Could you check a few things on this model? Use its own coordinates, in mm. Face numbers are marked on the shaded views. A direction names the side the tool comes from. Give positions to 0.01 mm unless a question says otherwise; leave off trailing zeros. Write each loop counter-clockwise with the first axis right and the second up, starting at its lowest first coordinate (ties: lowest second). Pieces come first, ordered by that corner, then holes. Notation, with made-up numbers: (47.5, 45) - (104.5, 45) arc R17 ccw to (104.5, 64) - close; hole circle Ø10 at (-14, -5.5). An arc over 180 degrees is marked (long way). Answer as CSV lines item,"result". Start each with the question number.
Q1. Imagine slicing it at A-A on z = 1.75. List the corners of the cut face in (x, y) for me, and give its area (3 significant figures).
Q2. Will these pins go through, and if not, where does the flat tip stop? pin 1 Ø1.5 at (x, z) = (52, 7.5) entering from -Y; pin 2 Ø3.5 at (y, z) = (6, 6) entering from -X; pin 3 Ø5 at (x, y) = (11.5, 38) entering from +Z.
Q3. Imagine slicing it at B-B on x = 33.5. List the corners of the cut face in (y, z) for me.
Q4. Imagine slicing it at C-C on y = 47.5. List the corners of the cut face in (x, z) for me, and give its area (3 significant figures).
Q5. Imagine slicing it at D-D on z = 8. List the corners of the cut face in (x, y) for me, and give its area (3 significant figures).
Q6. If I drill on line 1 along Y through (x, z) = (54.75, 6); line 2 along Z through (x, y) = (45.5, 21); line 3 along X through (y, z) = (11.5, 7), over which ranges is the centre line in solid material (lowest first)?
Q7. On a 3-axis mill with a long thin cutter (end or side, diameter ignored), from which of +Z, -Z, +X, -X, +Y, -Y can I reach the whole of each face in a straight line? I mean the marked faces 1 and 2. Say none if no direction works.
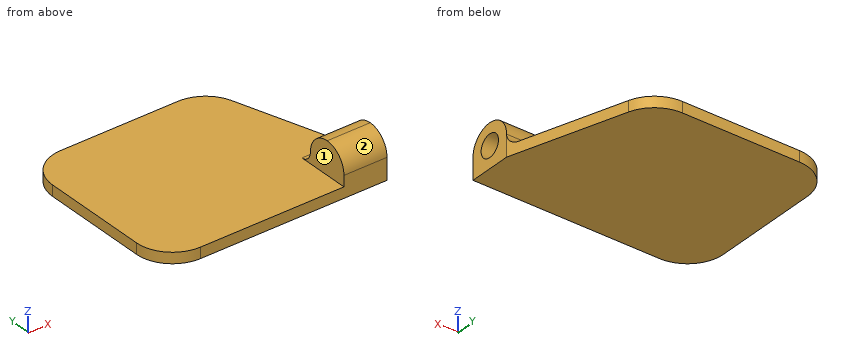
```python
from build123d import *

# Parameters (mm, degrees)
ESQUISSE1_W             = 50
ESQUISSE1_H             = 50
BOSS_EXTRU_1_DEPTH      = 3
BOSS_EXTRU_2_DEPTH      = 3
ESQUISSE3_W             = 12
ESQUISSE3_H             = 12
BOSS_EXTRU_3_DEPTH      = 9
ESQUISSE4_R             = 3.1
ENL_V_MAT_EXTRU_1_DEPTH = 10
CONG_1_R                = 6
CONG_2_R                = 3
CONG_3_R                = 10


with BuildPart() as part:
    # Esquisse1 → Boss.-Extru.1 (new body)
    with BuildSketch(Plane.XY):
        with Locations((25, 25)):
            Rectangle(ESQUISSE1_W, ESQUISSE1_H)
    extrude(amount=BOSS_EXTRU_1_DEPTH)

    # Esquisse2 → Boss.-Extru.2 (add)
    with BuildSketch(Plane.XY.offset(3)):
        Polygon((50, 0), (62, 0), (62, 12), (50, 50), align=None)
    extrude(amount=-BOSS_EXTRU_2_DEPTH)

    # Esquisse3 → Boss.-Extru.3 (add)
    with BuildSketch(Plane.XY.offset(3)):
        with Locations((56, 6)):
            Rectangle(ESQUISSE3_W, ESQUISSE3_H)
    extrude(amount=BOSS_EXTRU_3_DEPTH)

    # Esquisse4 → Enlèv. mat.-Extru.1 (cut)
    with BuildSketch(Plane(origin=(62, 0, 0), x_dir=(0, 0, -1), z_dir=(1, 0, 0))):
        with Locations((-6, 6)):
            Circle(ESQUISSE4_R)
    extrude(amount=-ENL_V_MAT_EXTRU_1_DEPTH, mode=Mode.SUBTRACT)

    # Congé1
    cong_1_edges = [part.edges().sort_by_distance(p)[0] for p in [
        (56, 0, 12),
        (56, 12, 12),
    ]]
    fillet(cong_1_edges, radius=CONG_1_R - 0.0001)  # a hair under: the kernel refuses the full size

    # Congé2
    cong_2_edges = [part.edges().sort_by_distance(p)[0] for p in [
        (56, 12, 3),
    ]]
    fillet(cong_2_edges, radius=CONG_2_R)

    # Congé3
    cong_3_edges = [part.edges().sort_by_distance(p)[0] for p in [
        (0, 0, 1.5),
        (0, 50, 1.5),
        (50, 50, 1.5),
    ]]
    fillet(cong_3_edges, radius=CONG_3_R)


solid = part.part
```
Conclusion:
1,outline,"(0, 10) arc R10 ccw to (10, 0) - (62, 0) - (62, 12) - (52.21, 43.01) arc R10 ccw to (42.67, 50) - (10, 50) arc R10 ccw to (0, 40) - close"
1,area,"2,820 mm^2"
2,pin 1,"y = 0.05"
2,pin 2,"x = 50"
2,pin 3,"z = 3"
3,outline,"(0, 0) - (50, 0) - (50, 3) - (0, 3) - close"
4,outline,"(3.39, 0) - (49.29, 0) - (49.29, 3) - (3.39, 3) - close"
4,area,"138 mm^2"
5,outline,"(50, 0.34) - (62, 0.34) - (62, 3.63) - (52, 3.63) - (52, 8.37) - (62, 8.37) - (62, 11.66) - (50, 11.66) - close"
5,area,"88.4 mm^2"
6,line 1,"0 to 2.9, 9.1 to 12"
6,line 2,"0 to 3"
6,line 3,"50 to 62"
7,face 1,"+Z, -X, +Y, -Y"
7,face 2,"+Z, +X, -X, -Y"
